Can you work these out from the model? Positions are in its coordinate system, mm. Face numbers are marked on the shaded views. A direction names the side the tool comes from. Give positions to 0.01 mm unless a question says otherwise; leave off trailing zeros. Loops run counter-clockwise (first coordinate to the right, second up) from the corner with the lowest first, then second, coordinate; pieces in that order, holes last. Notation, with made-up numbers: M 77.5,24 L 131.5,24 A22 cw 131.5,59 Z; hole C 76.25,-2 d1. An arc over 180 degrees is marked long. Use CSV: the item, a comma, the result in double quotes.
from build123d import *

# Parameters (mm, degrees)
F1_DEPTH = 14.5
F0_W     = 16.9
F0_H     = 21
F0_R     = 5.25
F0_W_2   = 7
F2_DEPTH = 17.2
F3_R     = 1.5
F4_DEPTH = 25


with BuildPart() as f1:
    # F0 (on Top) → F1 (new body)
    with BuildSketch(Plane.XY):
        with BuildLine():
            Line((7.4, -9.5), (-9.5, -9.5))
            ThreePointArc((-9.5, -9.5), (-9.879864, -12.835416), (-11, -16))
            Line((-11, -16), (-11, -30))
            Line((-11, -30), (-24, -30))
            Line((-24, -30), (-24, -37.5))
            Line((-24, -37.5), (30.9, -37.5))
            Line((30.9, -37.5), (30.9, -24.5))
            ThreePointArc((30.9, -24.5), (19.714686, -20.429433), (15, -9.5))
            Line((15, -9.5), (8, -9.5))
            Line((8, -9.5), (8, -15.040408))
            ThreePointArc((8, -15.040408), (14.24664, -18.024695), (7.4, -17))
            Line((7.4, -17), (7.4, -9.5))
        make_face()
    extrude(amount=F1_DEPTH)

    # F0 (on Top) → F2 (join)
    with BuildSketch(Plane.XY):
        with Locations((-1.05, 1)):
            Rectangle(F0_W, F0_H)
        Circle(F0_R, mode=Mode.SUBTRACT)
        with Locations((11.5, 1)):
            Rectangle(F0_W_2, F0_H)
    extrude(amount=F2_DEPTH)

    # F3 (on face) → F4 (cut)
    with BuildSketch(Plane.XY.offset(17.2)):
        with Locations((11, 0)):
            Circle(F3_R)
    extrude(amount=-F4_DEPTH, mode=Mode.SUBTRACT)


solid = f1.part
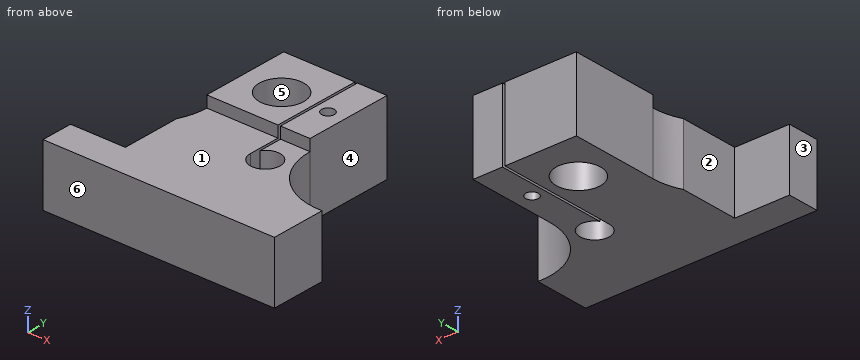
Q1. I want a section at B-B, the plane y = 8. Please give me the cut outline in (x, z).
Model answer:
outline,"M -9.5,0 L 7.4,0 L 7.4,17.2 L -9.5,17.2 Z; M 8,0 L 15,0 L 15,17.2 L 8,17.2 Z"
Q2. I want a section at A-A, the plane x = 0. Please give me the cut outline in (y, z).
Model answer:
outline,"M -37.5,0 L -5.25,0 L -5.25,17.2 L -9.5,17.2 L -9.5,14.5 L -37.5,14.5 Z; M 5.25,0 L 11.5,0 L 11.5,17.2 L 5.25,17.2 Z"
Q3. Please list where these lines run through material, in increasing order: L1, parallel to Y at x = 11, z = 6.5; L2, parallel to X at y = 8, z = 1.75; L3, parallel to X at y = 2, z = 10.25. Write a range as from..to.
Model answer:
L1,"-37.5..-20.5, -13.5..-1.5, 1.5..11.5"
L2,"-9.5..7.4, 8..15"
L3,"-9.5..-4.85, 4.85..7.4, 8..15"
Q4. I want a section at C-C, the plane y = 0. Please give me the cut outline in (x, z).
Model answer:
outline,"M -9.5,0 L -5.25,0 L -5.25,17.2 L -9.5,17.2 Z; M 5.25,0 L 7.4,0 L 7.4,17.2 L 5.25,17.2 Z; M 8,0 L 9.5,0 L 9.5,17.2 L 8,17.2 Z; M 12.5,0 L 15,0 L 15,17.2 L 12.5,17.2 Z"
Q5. I'm going to push flat-ended pins straight in: P1, Ø8.5, axis at x = 0, y = 0, coming from the -Z side; P2, Ø3, axis at y = -18, z = 12, coming from the -X side; P3, Ø0.8, axis at x = 11, z = 15.5, coming from the -Y side; P4, Ø11, axis at x = 10.9, y = -17, coming from the +Z side. Where does each tip first touch, or does it pass through?
Model answer:
P1,"through"
P2,"x = -11"
P3,"y = -9.5"
P4,"z = 14.5"
Q6. For the marked faces 1, 2 and 3, which set-ups out of +Z, -Z, +X, -X, +Y, -Y let a thin tool reach every point of the face, with its end or its side?
Model answer:
face 1,"+Z, +X, -X, -Y"
face 2,"+Z, -Z, -X, +Y"
face 3,"+Z, -Z, -X, +Y, -Y"
Q7. I want a section at D-D, the plane x = 11. Please give me the cut outline in (y, z).
Model answer:
outline,"M -37.5,0 L -20.5,0 L -20.5,14.5 L -37.5,14.5 Z; M -13.5,0 L -1.5,0 L -1.5,17.2 L -9.5,17.2 L -9.5,14.5 L -13.5,14.5 Z; M 1.5,0 L 11.5,0 L 11.5,17.2 L 1.5,17.2 Z"
Q8. If we mould it in two halves opening along X, with no side actions, what happens to the marked faces 4, 5 and 6? For each: released by +X, released by -X, zero draft, split by the parting line, or undercut.
Model answer:
face 4,"released by +X"
face 5,"undercut"
face 6,"zero draft"
